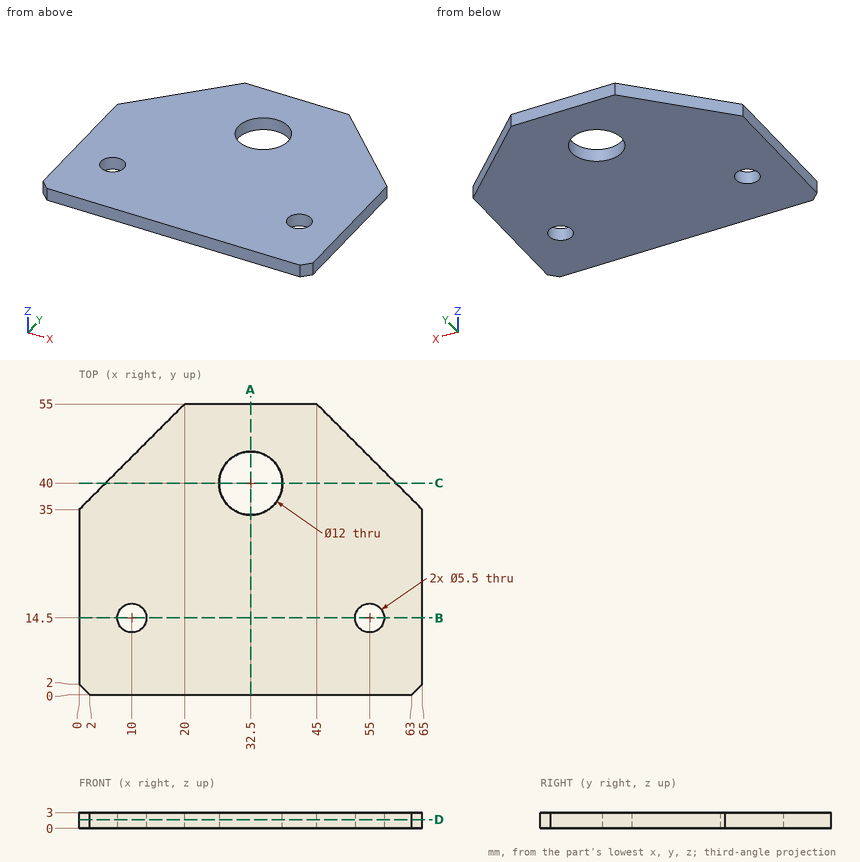
Here's the drawing with two shaded views (mm, measured from the low corner). I have some questions. Round coordinates to 2 decimals unless told otherwise and drop trailing zeros. Write each loop counter-clockwise with the first axis right and the second up, starting at its lowest first coordinate (ties: lowest second). Pieces come first, ordered by that corner, then holes.
(1) For pin 1 (6 mm diameter, centred on x = 34.5, y = 39.5, fed in from +Z), with a flat end and sliding along its axis, tell me the tip position at first contact or that it passes through.
Findings below:
pin 1: passes through
(2) Suppose I cut it at C-C on y = 40. Write out the boundary of the cut face in (x, z).
Findings below:
outline: (5, 0) - (26.5, 0) - (26.5, 3) - (5, 3) - close; (38.5, 0) - (60, 0) - (60, 3) - (38.5, 3) - close
(3) Suppose I cut it at B-B on y = 14.5. Write out the boundary of the cut face in (x, z).
Findings below:
outline: (0, 0) - (7.25, 0) - (7.25, 3) - (0, 3) - close; (12.75, 0) - (52.25, 0) - (52.25, 3) - (12.75, 3) - close; (57.75, 0) - (65, 0) - (65, 3) - (57.75, 3) - close
(4) Suppose I cut it at D-D on z = 1.65. Write out the boundary of the cut face in (x, y).
Findings below:
outline: (0, 2) - (2, 0) - (63, 0) - (65, 2) - (65, 35) - (45, 55) - (20, 55) - (0, 35) - close; hole circle Ø5.5 at (10, 14.5); hole circle Ø12 at (32.5, 40); hole circle Ø5.5 at (55, 14.5)
(5) Suppose I cut it at A-A on x = 32.5. Write out the boundary of the cut face in (y, z).
Findings below:
outline: (0, 0) - (34, 0) - (34, 3) - (0, 3) - close; (46, 0) - (55, 0) - (55, 3) - (46, 3) - close
(6) If I drill on probe 1 along Y at (x, z) = (10, 2.3); probe 2 along X at (y, z) = (17, 0.15); probe 3 along Y at (x, z) = (32.5, 2.3), over which ranges is the centre line in solid material (lowest first)?
Findings below:
probe 1: y = 0 to 11.75, 17.25 to 45
probe 2: x = 0 to 8.85, 11.15 to 53.85, 56.15 to 65
probe 3: y = 0 to 34, 46 to 55
